```python
from build123d import *

# Parameters (mm, degrees)
BOSS_EXTRUDE1_DEPTH = 2


with BuildPart() as part:
    # Sketch1 → Boss-Extrude1 (new body)
    with BuildSketch(Plane(origin=(0, 0, 0), x_dir=(1, 0, 0), z_dir=(0, 1, 0))):
        with BuildLine():
            Line((-23.335340856, 23.970044555), (-15.335340856, 23.970044555))
            Line((-15.335340856, 23.970044555), (-15.335340856, 47.670044555))
            ThreePointArc((-15.335340856, 47.670044555), (-9.335340856, 53.670044555), (-3.335340856, 47.670044555))
            Line((-3.335340856, 47.670044555), (-3.335340856, 23.970044555))
            Line((-3.335340856, 23.970044555), (6.664659144, 23.970044555))
            Line((6.664659144, 23.970044555), (6.664659144, 47.670044555))
            ThreePointArc((6.664659144, 47.670044555), (12.664659144, 53.670044555), (18.664659144, 47.670044555))
            Line((18.664659144, 47.670044555), (18.664659144, 23.970044555))
            Line((18.664659144, 23.970044555), (26.664659144, 23.970044555))
            Line((26.664659144, 23.970044555), (26.664659144, -16.029955445))
            Line((26.664659144, -16.029955445), (18.664659144, -16.029955445))
            Line((18.664659144, -16.029955445), (18.664659144, -39.729955445))
            ThreePointArc((18.664659144, -39.729955445), (12.664659144, -45.729955445), (6.664659144, -39.729955445))
            Line((6.664659144, -39.729955445), (6.664659144, -16.029955445))
            Line((6.664659144, -16.029955445), (-3.335340856, -16.029955445))
            Line((-3.335340856, -16.029955445), (-3.335340856, -39.729955445))
            ThreePointArc((-3.335340856, -39.729955445), (-9.335340856, -45.729955445), (-15.335340856, -39.729955445))
            Line((-15.335340856, -39.729955445), (-15.335340856, -16.029955445))
            Line((-15.335340856, -16.029955445), (-23.335340856, -16.029955445))
            Line((-23.335340856, -16.029955445), (-23.335340856, 23.970044555))
        make_face()
        with BuildLine():
            Line((9.514659144, 47.670044555), (9.514659144, 42.529492266))
            ThreePointArc((9.514659144, 42.529492266), (12.664659144, 39.379492266), (15.814659144, 42.529492266))
            Line((15.814659144, 42.529492266), (15.814659144, 47.670044555))
            ThreePointArc((15.814659144, 47.670044555), (12.664659144, 50.820044555), (9.514659144, 47.670044555))
        make_face(mode=Mode.SUBTRACT)
        with BuildLine():
            Line((-6.185340856, 47.670044555), (-6.185340856, 42.529492266))
            ThreePointArc((-6.185340856, 42.529492266), (-9.335340856, 39.379492266), (-12.485340856, 42.529492266))
            Line((-12.485340856, 42.529492266), (-12.485340856, 47.670044555))
            ThreePointArc((-12.485340856, 47.670044555), (-9.335340856, 50.820044555), (-6.185340856, 47.670044555))
        make_face(mode=Mode.SUBTRACT)
        with BuildLine():
            Line((9.514659144, -39.729955445), (9.514659144, -34.589403157))
            ThreePointArc((9.514659144, -34.589403157), (12.664659144, -31.439403157), (15.814659144, -34.589403157))
            Line((15.814659144, -34.589403157), (15.814659144, -39.729955445))
            ThreePointArc((15.814659144, -39.729955445), (12.664659144, -42.879955445), (9.514659144, -39.729955445))
        make_face(mode=Mode.SUBTRACT)
        with BuildLine():
            Line((-6.185340856, -39.729955445), (-6.185340856, -34.589403157))
            ThreePointArc((-6.185340856, -34.589403157), (-9.335340856, -31.439403157), (-12.485340856, -34.589403157))
            Line((-12.485340856, -34.589403157), (-12.485340856, -39.729955445))
            ThreePointArc((-12.485340856, -39.729955445), (-9.335340856, -42.879955445), (-6.185340856, -39.729955445))
        make_face(mode=Mode.SUBTRACT)
    extrude(amount=BOSS_EXTRUDE1_DEPTH)


solid = part.part
```
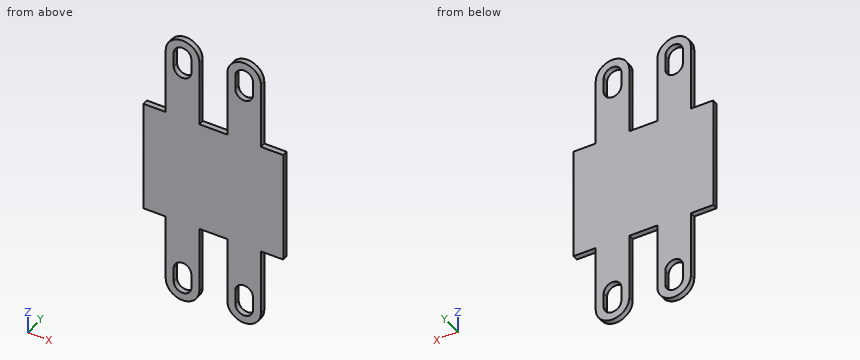
Verification items for the finished model (mm, model axes). Round coordinates to 2 decimals unless told otherwise and drop trailing zeros. Write each loop counter-clockwise with the first axis right and the second up, starting at its lowest first coordinate (ties: lowest second). Pieces come first, ordered by that corner, then holes.
1. Section check B-B on z = -38. Enter the section's corners in (x, y).
2. Section check C-C on y = 0.55. State how many separate pieces and enclosed holes the cut face has, plus the area to 3 significant figures.
3. Section check D-D on x = -18.5. Enter the section's corners in (y, z).
4. Scan lines: L1, parallel to X at y = 1.15, z = 36; L2, parallel to X at y = 1.35, z = 17; L3, parallel to X at y = 0.25, z = -42. Record each from-to range of solid material in increasing order.
5. Gauge pin test, flat ends, axial feed: P1, Ø0.6, axis at y = 1, z = 27, coming from the -X side; P2, Ø0.6, axis at y = 1.5, z = -44.5, coming from the +X side; P3, Ø1, axis at x = 7.5, y = 0.5, coming from the -Z side. Record the tip position at first contact, or that the pin passes through.
6. Section check A-A on z = 37. Enter the section's corners in (x, y), plus the area to 3 significant figures.
Answer:
1. outline: (-15.34, 0) - (-3.34, 0) - (-3.34, 2) - (-15.34, 2) - close; (6.66, 0) - (18.66, 0) - (18.66, 2) - (6.66, 2) - close
2. separate pieces: 1
2. enclosed holes: 4
2. area: 3,110 mm2
3. outline: (0, -23.97) - (2, -23.97) - (2, 16.03) - (0, 16.03) - close
4. L1: x = -15.34 to -12.49, -6.19 to -3.34, 6.66 to 9.51, 15.81 to 18.66
4. L2: x = -15.34 to -3.34, 6.66 to 18.66
4. L3: x = -15.34 to -12.44, -6.23 to -3.34, 6.66 to 9.56, 15.77 to 18.66
5. P1: stops at x = -15.34
5. P2: stops at x = 18.66
5. P3: stops at z = -51.44
6. outline: (-15.34, 0) - (-12.49, 0) - (-12.49, 2) - (-15.34, 2) - close; (-6.19, 0) - (-3.34, 0) - (-3.34, 2) - (-6.19, 2) - close; (6.66, 0) - (9.51, 0) - (9.51, 2) - (6.66, 2) - close; (15.81, 0) - (18.66, 0) - (18.66, 2) - (15.81, 2) - close
6. area: 22.8 mm2
